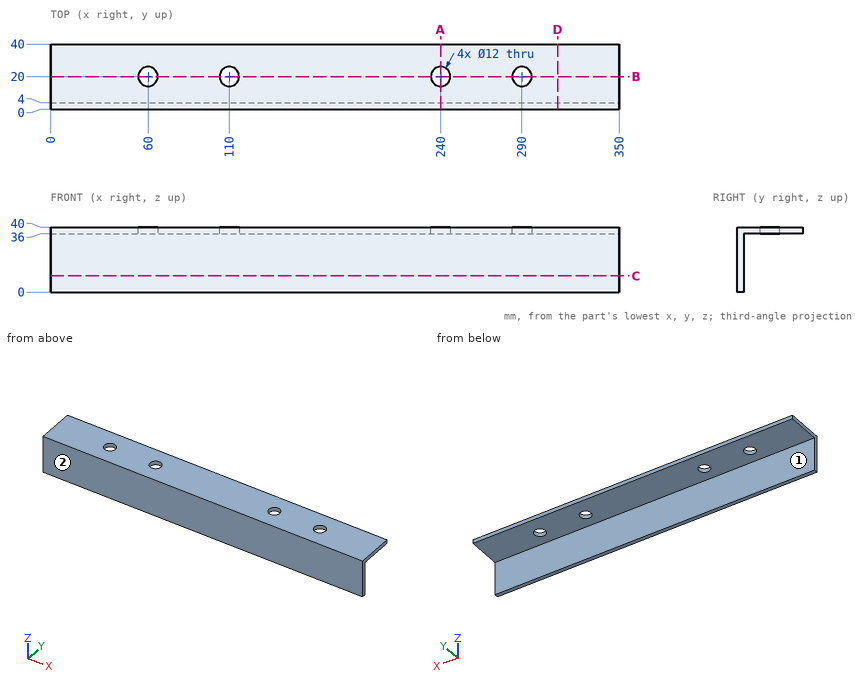
Here's the drawing with two shaded views (mm, measured from the low corner). I have some questions. A direction names the side the tool comes from. Coordinates: 2 decimals unless noted, no trailing zeros. Loops run counter-clockwise (first coordinate to the right, second up) from the corner with the lowest first, then second, coordinate; pieces in that order, holes last. Notation, with made-up numbers: (78.25, 76.25) -> (115.25, 76.25) arc R30 ccw to (115.25, 100.25) -> close; hole circle Ø6 at (46.5, -15.75). An arc over 180 degrees is marked (long way). Put each result on its own line as item: value. Start each with the question number.
Q1. I want a section at D-D (x = 312). Write out the boundary of the cut face in (y, z).
Q2. I'm going to push flat-ended pins straight in: P1, Ø9.5, axis at x = 240, y = 20, coming from the -Z side; P2, Ø12, axis at x = 99, y = 23, coming from the -Z side. Where does each tip first touch, or does it pass through?
Q3. If I drill on line 1 (Y direction, x = 110, z = 37); line 2 (Z direction, x = 53, y = 35); line 3 (Y direction, x = 179.5, z = 35), over which ranges is the centre line in solid material (lowest first)? Write a range as [from, to].
Q4. For the marked faces 1 and 2, which set-ups out of +Z, -Z, +X, -X, +Y, -Y let a thin tool reach every point of the face, with its end or its side?
Q5. I want a section at C-C (z = 10). Write out the boundary of the cut face in (x, y).
Q6. I want a section at B-B (y = 20). Write out the boundary of the cut face in (x, z).
Q7. I want a section at A-A (x = 240). Write out the boundary of the cut face in (y, z).
Taken from the geometry:
1. outline: (0, 0) -> (4, 0) -> (4, 36) -> (40, 36) -> (40, 40) -> (0, 40) -> close
2. P1: passes through
2. P2: stops at z = 36
3. line 1: y = [0, 14], [26, 40]
3. line 2: z = [36, 40]
3. line 3: y = [0, 4]
4. face 1: -Z, +X, -X, +Y
4. face 2: +Z, -Z, +X, -X, -Y
5. outline: (0, 0) -> (350, 0) -> (350, 4) -> (0, 4) -> close
6. outline: (0, 36) -> (54, 36) -> (54, 40) -> (0, 40) -> close; (66, 36) -> (104, 36) -> (104, 40) -> (66, 40) -> close; (116, 36) -> (234, 36) -> (234, 40) -> (116, 40) -> close; (246, 36) -> (284, 36) -> (284, 40) -> (246, 40) -> close; (296, 36) -> (350, 36) -> (350, 40) -> (296, 40) -> close
7. outline: (0, 0) -> (4, 0) -> (4, 36) -> (14, 36) -> (14, 40) -> (0, 40) -> close; (26, 36) -> (40, 36) -> (40, 40) -> (26, 40) -> close
